Verification items for the finished model (mm, model axes). A direction names the side the tool comes from. Give positions to 0.01 mm unless a question says otherwise; leave off trailing zeros. Order: outer loops, then holes, each group sorted by start corner. A loop starts at its lowest first (then second) coordinate and runs counter-clockwise, first axis right, second up. Notation, with made-up numbers: (82.25, 5) -> (120.25, 5) arc R26 ccw to (120.25, 22) -> close; hole circle Ø8 at (1.5, 62). An arc over 180 degrees is marked (long way). Write each question's results on one line, items separated by ' | '. Start each with the question number.
1. Set-up check for faces 5 (the face through (-3.47, -15.62, 31.44)), 6 (the face through (-34.11, -15.62, 3.47)), 7 (the face through (0.85, 27.85, -19.28)): record each of +Z, -Z, +X, -X, +Y, -Y from which the full face is reachable in a straight line by a thin tool's end or side.
2. Depth check by flat-ended pin: pin 1 Ø16 at (x, z) = (-0.5, 6) entering from -Y; pin 2 Ø4 at (x, y) = (35.5, 7.5) entering from -Z; pin 3 Ø1.5 at (x, y) = (-1.5, 33) entering from -Z. Enter the tip coordinate at first touch or a pass-through.
3. Mould release check, pull along Z, two halves, no side actions. Record for faces 1 (the face through (16.343, 10.269, -8.916)), 2 (the face through (27.846, 5.797, -18.409)), 3 (the face through (33.79, -15.62, 3.47)), 4 (the face through (-45.05, 16, -3)): +Z half, -Z half, draft (parallel to the pull), parting line (faces both ways), or undercut.
4. Cross-section at D-D, the plane x = -38.5. Enter the section's corners in (y, z), then the cut area to 3 significant figures.
5. Material ranges on L1, parallel to Y at x = 0, z = 31; L2, parallel to X at y = 0.5, z = 34; L3, parallel to Z at x = 0, y = -20, recorded low to high. Write a range as from..to.
from build123d import *

# Parameters (mm, degrees)
SKETCH_1_R               = 19.3
SKETCH_1_R_2             = 13.6
EXTRUDE_1_DEPTH          = 45.05
SKETCH_3_R               = 19.3
SKETCH_3_R_2             = 13.6
EXTRUDE_3_DEPTH          = 45.05
SKETCH_2_R               = 19.3
SKETCH_2_R_2             = 13.6
EXTRUDE_2_DEPTH          = 42.7
CUT_EXTRUDE_1_DEPTH      = 77.696121327
CUT_EXTRUDE_1_DEPTH_BACK = 77.696121327
SKETCH_1_13_R            = 13.6
CUT_EXTRUDE_START        = -19.3000001
CUT_EXTRUDE_2_OUTLINE_R  = 13.6
CUT_EXTRUDE_2_DEPTH      = 38.6000002
CUT_EXTRUDE_START_2      = 9.616652
SKETCH_2_8_R             = 13.6
CUT_EXTRUDE_3_DEPTH      = 9.683348
CUT_EXTRUDE_START_3      = -45.05
SKETCH_1_15_R            = 16
CUT_EXTRUDE_4_DEPTH      = 22.2
CUT_EXTRUDE_START_4      = 22.85
SKETCH_1_16_R            = 16
CUT_EXTRUDE_5_DEPTH      = 22.2
SKETCH_3_9_R             = 16
CUT_EXTRUDE_6_DEPTH      = 22.2
SKETCH_3_10_R            = 16
CUT_EXTRUDE_7_DEPTH      = 22.2
CUT_EXTRUDE_START_5      = 20.5
SKETCH_2_9_R             = 16
SKETCH_2_9_R_2           = 13.6
CUT_EXTRUDE_8_DEPTH      = 22.2


# Read off the part's stored shape, not the designer's step: 切除-拉伸2
with BuildPart() as part:
    # 草图1 → 凸台-拉伸1 (new, symmetric)
    with BuildSketch(Plane(origin=(0, 0, 0), x_dir=(1, 0, 0), z_dir=(0, 1, 0))):
        with Locations(Location((0, 0, 0), (0, 0, 270))):
            Circle(SKETCH_1_R)
        with Locations(Location((0, 0, 0), (0, 0, 270))):
            Circle(SKETCH_1_R_2, mode=Mode.SUBTRACT)
    extrude(amount=EXTRUDE_1_DEPTH, both=True)

    # 草图3 → 凸台-拉伸3 (add, symmetric)
    with BuildSketch(Plane(origin=(0, 0, 0), x_dir=(0, 0, -1), z_dir=(1, 0, 0))):
        Circle(SKETCH_3_R)
        with Locations(Location((0, 0, 0), (0, 0, 135.000000053))):
            Circle(SKETCH_3_R_2, mode=Mode.SUBTRACT)
    extrude(amount=EXTRUDE_3_DEPTH, both=True)

    # 草图2 → 凸台-拉伸2 (add)
    with BuildSketch(Plane.XY):
        with Locations(Location((0, 0, 0), (0, 0, 225))):
            Circle(SKETCH_2_R)
        with Locations(Location((0, 0, 0), (0, 0, 224.999996881))):
            Circle(SKETCH_2_R_2, mode=Mode.SUBTRACT)
    extrude(amount=EXTRUDE_2_DEPTH)

    # 草图1<13> → 切除-拉伸1 (cut, two sides: drawn at the far end of the back side and taken through both)
    with BuildSketch(Plane(origin=(0, 0, 0), x_dir=(1, 0, 0), z_dir=(0, 1, 0)).offset(-CUT_EXTRUDE_1_DEPTH_BACK)):
        with Locations(Location((0, 0, 0), (0, 0, 270))):
            Circle(SKETCH_1_13_R)
    extrude(amount=CUT_EXTRUDE_1_DEPTH + CUT_EXTRUDE_1_DEPTH_BACK, mode=Mode.SUBTRACT)

    # 切除-拉伸2 outline → 切除-拉伸2 (cut)
    with BuildSketch(Plane(origin=(0, 0, 0), x_dir=(0, 0, -1), z_dir=(1, 0, 0)).offset(CUT_EXTRUDE_START)):
        Circle(CUT_EXTRUDE_2_OUTLINE_R)
    extrude(amount=CUT_EXTRUDE_2_DEPTH, mode=Mode.SUBTRACT)

    # 草图2<8> → 切除-拉伸3 (cut)
    with BuildSketch(Plane.XY.offset(CUT_EXTRUDE_START_2)):
        with Locations(Location((0, 0, 0), (0, 0, 225))):
            Circle(SKETCH_2_8_R)
    extrude(amount=CUT_EXTRUDE_3_DEPTH, mode=Mode.SUBTRACT)

    # 草图1<15> → 切除-拉伸4 (cut)
    with BuildSketch(Plane(origin=(0, 0, 0), x_dir=(1, 0, 0), z_dir=(0, 1, 0)).offset(CUT_EXTRUDE_START_3)):
        with Locations(Location((0, 0, 0), (0, 0, 270))):
            Circle(SKETCH_1_15_R)
    extrude(amount=CUT_EXTRUDE_4_DEPTH, mode=Mode.SUBTRACT)

    # 草图1<16> → 切除-拉伸5 (cut)
    with BuildSketch(Plane(origin=(0, 0, 0), x_dir=(1, 0, 0), z_dir=(0, 1, 0)).offset(CUT_EXTRUDE_START_4)):
        with Locations(Location((0, 0, 0), (0, 0, 270))):
            Circle(SKETCH_1_16_R)
    extrude(amount=CUT_EXTRUDE_5_DEPTH, mode=Mode.SUBTRACT)

    # 草图3<9> → 切除-拉伸6 (cut)
    with BuildSketch(Plane(origin=(0, 0, 0), x_dir=(0, 0, -1), z_dir=(1, 0, 0)).offset(CUT_EXTRUDE_START_3)):
        Circle(SKETCH_3_9_R)
    extrude(amount=CUT_EXTRUDE_6_DEPTH, mode=Mode.SUBTRACT)

    # 草图3<10> → 切除-拉伸7 (cut)
    with BuildSketch(Plane(origin=(0, 0, 0), x_dir=(0, 0, -1), z_dir=(1, 0, 0)).offset(CUT_EXTRUDE_START_4)):
        Circle(SKETCH_3_10_R)
    extrude(amount=CUT_EXTRUDE_7_DEPTH, mode=Mode.SUBTRACT)

    # 草图2<9> → 切除-拉伸8 (cut)
    with BuildSketch(Plane.XY.offset(CUT_EXTRUDE_START_5)):
        Circle(SKETCH_2_9_R)
        with Locations(Location((0, 0, 0), (0, 0, 225))):
            Circle(SKETCH_2_9_R_2, mode=Mode.SUBTRACT)
    extrude(amount=CUT_EXTRUDE_8_DEPTH, mode=Mode.SUBTRACT)


solid = part.part
Results below:
1) face 5: +Z | face 6: -X | face 7: +Y
2) pin 1: stops at y = -22.85 | pin 2: stops at z = -18.5 | pin 3: stops at z = -19.29
3) face 1: undercut | face 2: parting line | face 3: undercut | face 4: draft
4) outline: circle Ø38.6 at (0, 0); hole circle Ø32 at (0, 0) | area: 366 mm²
5) L1: y = -19.3..-16, 16..19.3 | L2: x = -19.29..-15.99, 15.99..19.29 | L3: z = -19.3..-13.6, 13.6..19.3
